Autodesk Inventor part; units mm, degrees
ref_plane "YZ Plane" through (0, 0, 0) normal (1, 0, 0) x (0, 1, 0)
ref_plane "XZ Plane" through (0, 0, 0) normal (0, 1, 0) x (-1, 0, 0)
ref_plane "XY Plane" through (0, 0, 0) normal (0, 0, 1) x (1, 0, 0)
sketch "Sketch1" plane through (0, 0, 0) normal (0, 0, 1) x (1, 0, 0)
  line L0 (0, 0) -> (12, 0) construction
  line L1 (12, 0) -> (12, 38)
  line L2 (12, 38) -> (0, 38) construction
  line L3 (0, 38) -> (0, 0)
  arc A0 (12, 38) -> (0, 38) centre (6, 38) ccw
  arc A1 (0, 0) -> (12, 0) centre (6, 0) ccw
  circle A2 centre (6, 38) radius 1.5
  circle A3 centre (6, 0) radius 2.5
  circle A4 centre (6, 20) radius 1.5
  circle A5 centre (6, 28) radius 1.5
  dimension "d0" = 12
  dimension "d1" = 38
  dimension "d2" = 3
  dimension "d3" = 5
  dimension "d6" = 3
  dimension "d7" = 20
  dimension "d8" = 3
  dimension "d9" = 10
extrude "Extrusion1" add sketch "Sketch1" along normal blind 4
properties part number "z axis arm2"
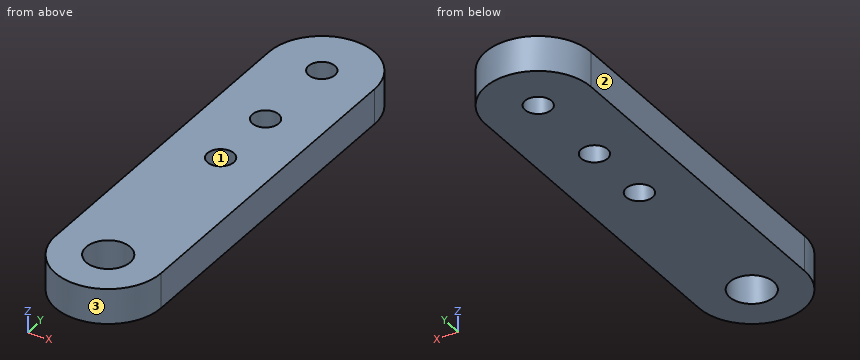
Could you check a few things on this model? Use its own coordinates, in mm. Face numbers are marked on the shaded views. Round coordinates to 2 decimals unless told otherwise and drop trailing zeros. Write each loop counter-clockwise with the first axis right and the second up, starting at its lowest first coordinate (ties: lowest second). Pieces come first, ordered by that corner, then holes. Notation, with made-up numbers: (-12, -25.5) - (23, -25.5) arc R17 ccw to (23, -15.5) - close; hole circle Ø2 at (-4.5, 73.5). An arc over 180 degrees is marked (long way). Use a Markdown table: item, result.
Q1. Please list where these lines run through material, in increasing order: L1, parallel to Y at x = 6, z = 2.5; L2, parallel to Y at x = 8, z = 2.4; L3, parallel to Y at x = 4.75, z = 1.05.
Output values:
| item | result |
|---|---|
| L1 | -6 to -2.5, 2.5 to 18.5, 21.5 to 26.5, 29.5 to 36.5, 39.5 to 44 |
| L2 | -5.66 to -1.5, 1.5 to 43.66 |
| L3 | -5.87 to -2.17, 2.17 to 19.17, 20.83 to 27.17, 28.83 to 37.17, 38.83 to 43.87 |
Q2. I want a section at D-D (x = 10.5). List the corners of the cut face in (y, z) for me.
Output values:
| item | result |
|---|---|
| outline | (-3.97, 0) - (41.97, 0) - (41.97, 4) - (-3.97, 4) - close |
Q3. Thinking about a two-plate mould opening in X: for the marked faces 1, 2 and 3, which applies, released by +X, released by -X, zero draft, split by the parting line, or undercut?
Output values:
| item | result |
|---|---|
| face 1 | undercut |
| face 2 | released by -X |
| face 3 | split by the parting line |
Q4. I want a section at B-B (x = 6). List the corners of the cut face in (y, z) for me.
Output values:
| item | result |
|---|---|
| outline | (-6, 0) - (-2.5, 0) - (-2.5, 4) - (-6, 4) - close; (2.5, 0) - (18.5, 0) - (18.5, 4) - (2.5, 4) - close; (21.5, 0) - (26.5, 0) - (26.5, 4) - (21.5, 4) - close; (29.5, 0) - (36.5, 0) - (36.5, 4) - (29.5, 4) - close; (39.5, 0) - (44, 0) - (44, 4) - (39.5, 4) - close |
Q5. I want a section at C-C (z = 0.6). List the corners of the cut face in (x, y) for me.
Output values:
| item | result |
|---|---|
| outline | (0, 0) arc R6 ccw to (12, 0) - (12, 38) arc R6 ccw to (0, 38) - close; hole circle Ø5 at (6, 0); hole circle Ø3 at (6, 20); hole circle Ø3 at (6, 28); hole circle Ø3 at (6, 38) |
Q6. I want a section at A-A (y = 20). List the corners of the cut face in (x, z) for me, plus the area to 3 significant figures.
Output values:
| item | result |
|---|---|
| outline | (0, 0) - (4.5, 0) - (4.5, 4) - (0, 4) - close; (7.5, 0) - (12, 0) - (12, 4) - (7.5, 4) - close |
| area | 36.0 mm2 |
Q7. For pin 1 (6.5 mm diameter, centred on x = 6, y = 0, fed in from +Z); pin 2 (1.5 mm diameter, centred on x = 4, z = 2, fed in from -Y), each with a flat end and sliding along its axis, tell me the tip position at first contact or that it passes through.
Output values:
| item | result |
|---|---|
| pin 1 | z = 4 |
| pin 2 | y = -5.87 |
